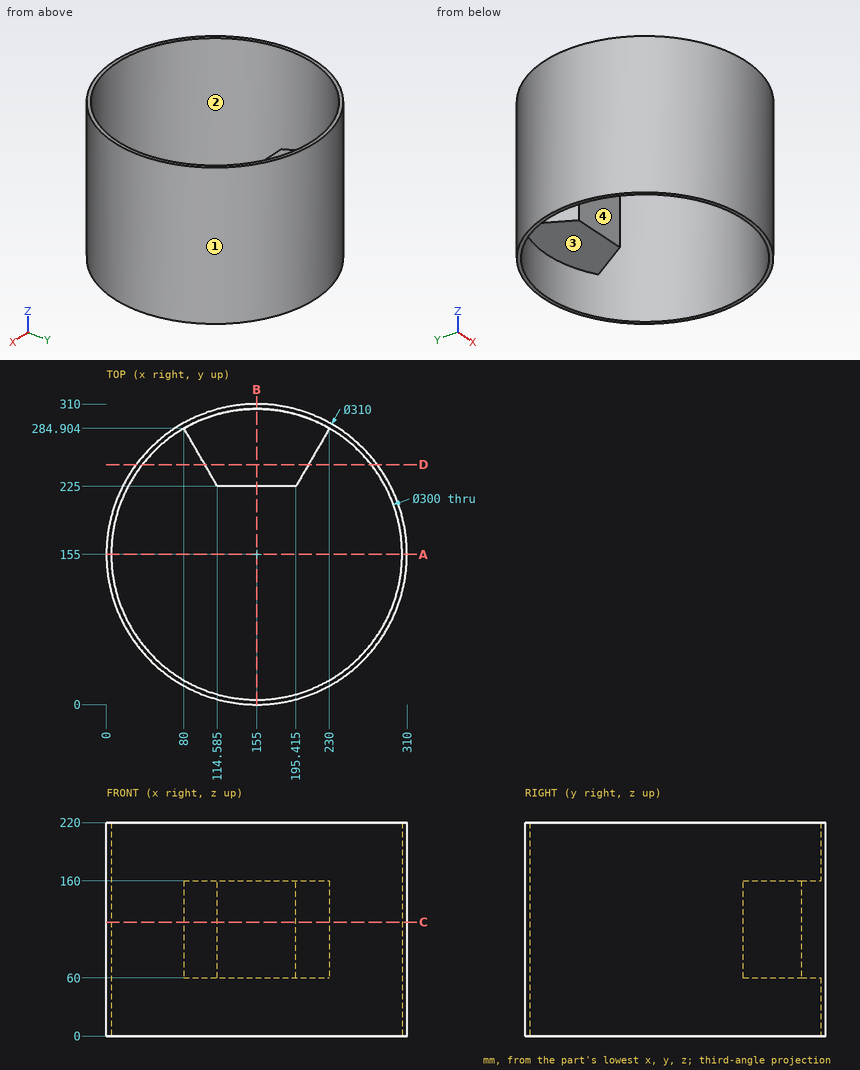
Design review of the part shown in the three views and the two pictorial views. Dimensions are in mm from the part's minimum x, y and z. A direction names the side the tool comes from. Give positions to 0.01 mm unless a question says otherwise; leave off trailing zeros. Loops run counter-clockwise (first coordinate to the right, second up) from the corner with the lowest first, then second, coordinate; pieces in that order, holes last. Notation, with made-up numbers: M 50,1 L 64,1 A31 ccw 64,30 Z; hole C 69,57.5 d1. An arc over 180 degrees is marked long. Answer as a JSON object with one key per item and string values.
Item 1: Mouldability with a two-part tool opening along Y and no side actions: class the marked faces 1 and 2 as pulls with the +Y half, pulls with the -Y half, needs draft (parallel to the pull), parting line crosses it, or undercut.
Output values:
{"face 1": "parting line crosses it", "face 2": "undercut"}
Item 2: Wall thickness on line 1 along Y through (x, z) = (155, 122); line 2 along Z through (x, y) = (165, 246); line 3 along Y through (x, z) = (105, 64.5) (1 decimal): over which ranges is each line inside the solid? List them lowest first.
Output values:
{"line 1": "y = 0 to 5, 225 to 310", "line 2": "z = 60 to 160", "line 3": "y = 8.3 to 13.6, 241.6 to 301.7"}
Item 3: We need section A-A (y = 155). State the section outline as (x, z) points, and give its area (3 significant figures).
Output values:
{"outline": "M 0,0 L 5,0 L 5,220 L 0,220 Z; M 305,0 L 310,0 L 310,220 L 305,220 Z", "area": "2,200 mm2"}
Item 4: Machinability: for the marked faces 3 and 4, which of the approach directions +Z, -Z, +X, -X, +Y, -Y give a long, thin tool a straight path to every point of the face, cutting with its end or side? Answer none if there is none.
Output values:
{"face 3": "-Z", "face 4": "+Z, -Z"}
Item 5: For P1, Ø1, axis at y = 87, z = 106, coming from the +X side; P2, Ø3, axis at x = 103, z = 149.5, coming from the -Y side; P3, Ø1, axis at y = 182.5, z = 125.5, coming from the -X side, all flat-tipped, find the tip position at first contact; note any pin that passes through.
Output values:
{"P1": "stops at x = 294.53", "P2": "stops at y = 8.46", "P3": "stops at x = 2.37"}
Item 6: We need section D-D (y = 247.5). State the section outline as (x, z) points (1 decimal).
Output values:
{"outline": "M 30.6,0 L 36.9,0 L 36.9,220 L 30.6,220 Z; M 101.6,60 L 208.4,60 L 208.4,160 L 101.6,160 Z; M 273.1,0 L 279.4,0 L 279.4,220 L 273.1,220 Z"}
Item 7: We need section B-B (x = 155). State the section outline as (y, z) points, and give its area (3 significant figures).
Output values:
{"outline": "M 0,0 L 5,0 L 5,220 L 0,220 Z; M 225,60 L 305,60 L 305,0 L 310,0 L 310,220 L 305,220 L 305,160 L 225,160 Z", "area": "10,200 mm2"}
Item 8: We need section C-C (z = 117.5). State the section outline as (x, y) points (1 decimal), and give its area (3 significant figures).
Output values:
{"outline": "C 155,155 d310; hole M 80,284.9 A150 ccw long 230,284.9 L 195.4,225 L 114.6,225 Z", "area": "13,700 mm2"}
